Could you check a few things on this model? Use its own coordinates, in mm. A direction names the side the tool comes from. Give positions to 0.01 mm unless a question says otherwise; leave off trailing zeros. Loops run counter-clockwise (first coordinate to the right, second up) from the corner with the lowest first, then second, coordinate; pieces in that order, holes last.
1. Thinking about a two-plate mould opening in X: for faces 1 (the flat face through (0, 0, 0)), 2 (the flat face through (0, -80.01, 0)), 3 (the flat face through (3.81, -3, 16)), which applies, +X half, -X half, draft (parallel to the pull), parting line (faces both ways), or undercut?
2. Imagine slicing it at C-C (y = -77). List the corners of the cut face in (x, z) for me.
3. For P1, Ø4, axis at x = 7.5, y = -69.5, coming from the +Z side; P2, Ø1.3, axis at y = -81.5, z = -0.5, coming from the +X side; P3, Ø3, axis at y = -4, z = 14.5, coming from the -X side; P4, Ø10, axis at x = 0, z = 4, coming from the +Y side, each with a flat end and sliding along its axis, tell me the tip position at first contact or that it passes through.
4. Imagine slicing it at A-A (x = 0). List the corners of the cut face in (y, z) for me, plus the area to 3 significant figures.
5. I need wall thicknesses on line 1 along Y through (x, z) = (10.5, -7); line 2 along Z through (x, y) = (0, -37); line 3 along Y through (x, z) = (0.75, 0). Which ranges of each line are inside material? Lowest first, please.
6. Imagine slicing it at D-D (z = 8). List the corners of the cut face in (x, y) for me, plus the area to 3 significant figures.
7. For faces 4 (the cylindrical face through (-0.5, -3.13, -12.69)), 5 (the flat face through (-1.27, -81, 0)), 6 (the flat face through (-3.81, -3, 16)), 7 (the flat face through (2, -82.55, 0)), 8 (the cylindrical face through (3.52, -76.29, -1.46)), which set-ups out of +Z, -Z, +X, -X, +Y, -Y let a thin tool reach every point of the face, with its end or its side?
8. Imagine slicing it at B-B (z = 0). List the corners of the cut face in (x, y) for me.
```python
from build123d import *

# Parameters (mm, degrees)
F1_DEPTH = 6.35
F2_R     = 6.35
F3_DEPTH = 76.2
F4_R     = 6.35
F4_R_2   = 3.81
F5_DEPTH = 12.7
F6_W     = 2.54
F6_H     = 25.4
F7_DEPTH = 2.54


with BuildPart() as f1:
    # F0 (on Front) → F1 (new body)
    with BuildSketch(Plane.XZ):
        with BuildLine():
            Line((-3.81, 19.05), (-3.81, 12.115028))
            ThreePointArc((-3.81, 12.115028), (0, -12.7), (3.81, 12.115028))
            Line((3.81, 12.115028), (3.81, 19.05))
            Line((3.81, 19.05), (-3.81, 19.05))
        make_face()
    extrude(amount=F1_DEPTH)

    # F2 (on face) → F3 (join)
    with BuildSketch(Plane.XZ.offset(6.35)):
        Circle(F2_R)
    extrude(amount=F3_DEPTH)

    # F4 (on face) → F5 (cut)
    with BuildSketch(Plane.XZ.offset(82.55)):
        Circle(F4_R)
        Circle(F4_R_2, mode=Mode.SUBTRACT)
    extrude(amount=-F5_DEPTH, mode=Mode.SUBTRACT)

    # F6 (on face) → F7 (cut)
    with BuildSketch(Plane.XZ.offset(82.55)):
        Rectangle(F6_W, F6_H)
    extrude(amount=-F7_DEPTH, mode=Mode.SUBTRACT)


solid = f1.part
```
Derived:
1. face 1: draft
1. face 2: undercut
1. face 3: +X half
2. outline: circle Ø7.62 at (0, 0)
3. P1: stops at z = 3.17
3. P2: stops at x = 3.81
3. P3: stops at x = -3.81
3. P4: stops at y = 0
4. outline: (-80.01, -3.81) - (-69.85, -3.81) - (-69.85, -6.35) - (-6.35, -6.35) - (-6.35, -12.7) - (0, -12.7) - (0, 19.05) - (-6.35, 19.05) - (-6.35, 6.35) - (-69.85, 6.35) - (-69.85, 3.81) - (-80.01, 3.81) - close
4. area: 1,090 mm2
5. line 1: y = -6.35 to 0
5. line 2: z = -6.35 to 6.35
5. line 3: y = -80.01 to 0
6. outline: (-9.86, -6.35) - (9.86, -6.35) - (9.86, 0) - (-9.86, 0) - close
6. area: 125 mm2
7. face 4: +Y, -Y
7. face 5: +Z, -Z, -Y
7. face 6: +Z, -X, +Y, -Y
7. face 7: +Z, -Z, +X, -X, -Y
7. face 8: -Y
8. outline: (-12.7, -6.35) - (-6.35, -6.35) - (-6.35, -69.85) - (-3.81, -69.85) - (-3.81, -82.55) - (-1.27, -82.55) - (-1.27, -80.01) - (1.27, -80.01) - (1.27, -82.55) - (3.81, -82.55) - (3.81, -69.85) - (6.35, -69.85) - (6.35, -6.35) - (12.7, -6.35) - (12.7, 0) - (-12.7, 0) - close
